```python
from build123d import *

# Parameters (mm, degrees)
F0_W        = 125
F0_H        = 100
F1_DEPTH    = 25
F2_T        = -2.5
F3_T1_DEPTH = 95
F3_T3_DEPTH = 120
F3_T5_DEPTH = 170
F3_T7_DEPTH = 145


# Not quite as in the source:
# - a fillet or chamfer that OpenCascade refuses, or shapes differently, is made with other operations: its cross-section is extruded or revolved along the edge and cut away or added


with BuildPart() as f1:
    # F0 (on Top) → F1 (new body)
    with BuildSketch(Plane.XY):
        with Locations((62.5, 50)):
            Rectangle(F0_W, F0_H)
    extrude(amount=F1_DEPTH)

    # F2
    f2_openings = [f1.faces().sort_by_distance(p)[0] for p in [
        (62.5, 50, 25),
    ]]
    offset(amount=F2_T, openings=f2_openings)

    # F3: fillet of radius 9 on 10 edges, made by hand

    # F3_s2 → F3_t1 (join)
    with BuildSketch(Plane.XZ.offset(-97.5)):
        with BuildLine():
            ThreePointArc((2.5, 11.5), (5.1360389693, 5.1360389693), (11.5, 2.5))
            Line((11.5, 2.5), (2.5, 2.5))
            Line((2.5, 2.5), (2.5, 11.5))
        make_face()
        with BuildLine():
            ThreePointArc((122.5, 11.5), (119.8639610307, 5.1360389693), (113.5, 2.5))
            Line((113.5, 2.5), (122.5, 2.5))
            Line((122.5, 2.5), (122.5, 11.5))
        make_face()
    extrude(amount=F3_T1_DEPTH)

    # F3_s4 → F3_t3 (join)
    with BuildSketch(Plane.YZ.offset(2.5)):
        with BuildLine():
            ThreePointArc((2.5, 11.5), (5.1360389693, 5.1360389693), (11.5, 2.5))
            Line((11.5, 2.5), (2.5, 2.5))
            Line((2.5, 2.5), (2.5, 11.5))
        make_face()
        with BuildLine():
            ThreePointArc((97.5, 11.5), (94.8639610307, 5.1360389693), (88.5, 2.5))
            Line((88.5, 2.5), (97.5, 2.5))
            Line((97.5, 2.5), (97.5, 11.5))
        make_face()
    extrude(amount=F3_T3_DEPTH)

    # F3_s6 → F3_t5 (cut)
    with BuildSketch(Plane.YZ.offset(-22.5)):
        with BuildLine():
            ThreePointArc((0, 16), (2.6360389693, 22.3639610307), (9, 25))
            Line((9, 25), (0, 25))
            Line((0, 25), (0, 16))
        make_face()
        with BuildLine():
            ThreePointArc((0, 9), (2.6360389693, 2.6360389693), (9, 0))
            Line((9, 0), (0, 0))
            Line((0, 0), (0, 9))
        make_face()
        with BuildLine():
            ThreePointArc((100, 16), (97.3639610307, 22.3639610307), (91, 25))
            Line((91, 25), (100, 25))
            Line((100, 25), (100, 16))
        make_face()
    extrude(amount=F3_T5_DEPTH, mode=Mode.SUBTRACT)

    # F3_s8 → F3_t7 (cut)
    with BuildSketch(Plane.XZ.offset(-122.5)):
        with BuildLine():
            ThreePointArc((116, 0), (122.3639610307, 2.6360389693), (125, 9))
            Line((125, 9), (125, 0))
            Line((125, 0), (116, 0))
        make_face()
        with BuildLine():
            ThreePointArc((116, 25), (122.3639610307, 22.3639610307), (125, 16))
            Line((125, 16), (125, 25))
            Line((125, 25), (116, 25))
        make_face()
        with BuildLine():
            ThreePointArc((0, 16), (2.6360389693, 22.3639610307), (9, 25))
            Line((9, 25), (0, 25))
            Line((0, 25), (0, 16))
        make_face()
    extrude(amount=F3_T7_DEPTH, mode=Mode.SUBTRACT)


solid = f1.part
```
Verification items for the finished model (mm, model axes). A direction names the side the tool comes from. Coordinates: 2 decimals unless noted, no trailing zeros. Write each loop counter-clockwise with the first axis right and the second up, starting at its lowest first coordinate (ties: lowest second). Pieces come first, ordered by that corner, then holes. Notation, with made-up numbers: M 41.25,-2 L 73.25,-2 A19 ccw 73.25,32 Z; hole C 24,-5.5 d11. An arc over 180 degrees is marked long. Answer as a JSON object with one key per item and string values. Group by question number.
(1) Cross-section at A-A, the plane x = 74.5. Record the cut outline in (y, z).
(2) Cross-section at C-C, the plane z = 7. Record the cut outline in (x, y), and give its area (3 significant figures).
(3) Gauge pin test, flat ends, axial feed: pin 1 (1.5 mm diameter, centred on x = 14.5, y = 38, fed in from +Z); pin 2 (4 mm diameter, centred on x = 112, y = 87.5, fed in from +Z). Record the tip position at first contact, or that the pin passes through.
(4) Material ranges on line 1 (X direction, y = 46.5, z = 14.25); line 2 (Y direction, x = 87.5, z = 16.25); line 3 (Y direction, x = 115.5, z = 20.5), recorded low to high.
(5) Cross-section at B-B, the plane y = 58. Record the cut outline in (x, z), and give its area (3 significant figures).
(6) Tool access check on faces 4 (the face through (61.63, 99.37, 19.31)), 5 (the face through (119.934, 50.665, 5.206)). Record the directions out of +Z, -Z, +X, -X, +Y, -Y that give a thin tool (end or side, any length) a straight path to the whole face; none if there is none.
(7) Release check for a two-part mould opening along Y. For faces 1 (the face through (62, 100, 8)), 2 (the face through (61.66, 94.934, 5.206)), 3 (the face through (122.294, 50.7, 2.566)) record: +Y half, -Y half, draft (parallel to the pull), parting line (faces both ways), or undercut.
Reply:
{
 "1": {"outline": "M 0,9 A9 ccw 9,0 L 100,0 L 100,16 A9 ccw 97.5,22.22 L 97.5,11.5 A9 cw 88.5,2.5 L 11.5,2.5 A9 cw 2.5,11.5 L 2.5,22.22 A9 ccw 0,16 Z"},
 "2": {"outline": "M 0,0.23 L 124.77,0.23 L 124.77,100 L 0,100 Z; hole M 3.71,3.71 L 121.29,3.71 L 121.29,96.29 L 3.71,96.29 Z", "area": "1,560 mm²"},
 "3": {"pin 1": "z = 2.5", "pin 2": "z = 2.56"},
 "4": {"line 1": "0 to 2.5, 122.5 to 125", "line 2": "0 to 2.5, 97.5 to 100", "line 3": "1.21 to 2.5, 97.5 to 98.79"},
 "5": {"outline": "M 0,0 L 116,0 A9 ccw 125,9 L 125,16 A9 ccw 122.5,22.22 L 122.5,11.5 A9 cw 113.5,2.5 L 11.5,2.5 A9 cw 2.5,11.5 L 2.5,22.22 A9 ccw 0,16 Z", "area": "419 mm²"},
 "6": {"face 4": "+Z, +X, -X, +Y", "face 5": "+Z"},
 "7": {"face 1": "+Y half", "face 2": "undercut", "face 3": "draft"}
}
